from build123d import *

# Parameters (mm, degrees)
SKETCH1_R              = 6.35
SKETCH1_R_2            = 11.1125
BOSS_EXTRUDE1_DEPTH    = 6.35
F_10_CLEARANCE_HOLE1_D = 4.9784


with BuildPart() as part:
    # Sketch1 → Boss-Extrude1 (new body)
    with BuildSketch(Plane(origin=(0, 0, 0), x_dir=(0, 0, -1), z_dir=(1, 0, 0))):
        with BuildLine():
            Line((-25.748192037, 52.738776596), (-10.728413349, -2.896343085))
            ThreePointArc((-10.728413349, -2.896343085), (0, -11.1125), (10.728413349, -2.896343085))
            Line((10.728413349, -2.896343085), (25.748192037, 52.738776596))
            ThreePointArc((25.748192037, 52.738776596), (26.438543659, 56.183961041), (26.67, 59.69))
            Line((26.67, 59.69), (26.67, 100.96397257))
            Line((26.67, 100.96397257), (-26.67, 100.96397257))
            Line((-26.67, 100.96397257), (-26.67, 59.69))
            ThreePointArc((-26.67, 59.69), (-26.438543659, 56.183961041), (-25.748192037, 52.738776596))
        make_face()
        Circle(SKETCH1_R, mode=Mode.SUBTRACT)
        with Locations((0, 59.69)):
            Circle(SKETCH1_R_2, mode=Mode.SUBTRACT)
    extrude(amount=BOSS_EXTRUDE1_DEPTH)

    # #10 Clearance Hole1 (through all)
    with Locations(Plane.ZY):
        with Locations((20.32, 96.20147257), (-20.32, 96.20147257)):
            Hole(F_10_CLEARANCE_HOLE1_D / 2)


solid = part.part
Check sheet for the modelled part. Datum: model origin and axes. Units: mm. Give positions to 0.01 mm unless a question says otherwise; leave off trailing zeros. Loops run counter-clockwise (first coordinate to the right, second up) from the corner with the lowest first, then second, coordinate; pieces in that order, holes last. Notation, with made-up numbers: M 44,40 L 73,40 A29 ccw 73,78 Z; hole C 51,56 d7. An arc over 180 degrees is marked long. Use a Markdown table: item, result. Add a question column.
Q1. Sectioned sample at C-C, the plane x = 4.75. Give the number of separate pieces and of enclosed holes in the cut face, then the cut area to 3 significant figures.
Q2. Sectioned sample at B-B, the plane z = -5. Record the cut outline in (x, y).
Q3. Sectioned sample at D-D, the plane z = -20.32. Record the cut outline in (x, y), then the cut area to 3 significant figures.
Q4. Sectioned sample at A-A, the plane z = 9. Record the cut outline in (x, y), then the cut area to 3 significant figures.
Q5. Mould release check, pull along Z, two halves, no side actions. Record for faces 1 (the cylindrical face through (3.13, -11.11, 0.2)), 2 (the cylindrical face through (3.219, 93.993, -21.469)), 3 (the flat face through (3, 81, 26.67)), 4 (the cylindrical face through (3.131, 49.831, -5.128)): pulls with the +Z half, pulls with the -Z half, needs draft (parallel to the pull), parting line crosses it, or undercut.
Q6. Scan lines: line 1 along Y through (x, z) = (1, -4); line 2 along Z through (x, y) = (3, 95); line 3 along Z through (x, y) = (6, 23.5). Record each from-to range of solid material in increasing order. Write a range as [from, to].
Q7. Go/stop test with flat-tipped pins: pin 1 (4 mm diameter, centred on y = 96.2, z = 20.32, fed in from -X); pin 2 (1.5 mm diameter, centred on x = 5, z = 1.5, fed in from -Y); pin 3 (10 mm diameter, centred on y = 19, z = 17, fed in from +X); pin 4 (3 mm diameter, centred on x = 4.5, y = 55.5, fed in from +Z). Record where each tip stops, or that it passes through.
Verdict:
| question | item | result |
|---|---|---|
| 1 | separate pieces | 1 |
| 1 | enclosed holes | 4 |
| 1 | area | 4,170 mm^2 |
| 2 | outline | M 0,-9.92 L 6.35,-9.92 L 6.35,-3.91 L 0,-3.91 Z; M 0,3.91 L 6.35,3.91 L 6.35,49.77 L 0,49.77 Z; M 0,69.61 L 6.35,69.61 L 6.35,100.96 L 0,100.96 Z |
| 3 | outline | M 0,32.63 L 6.35,32.63 L 6.35,93.71 L 0,93.71 Z; M 0,98.69 L 6.35,98.69 L 6.35,100.96 L 0,100.96 Z |
| 3 | area | 402 mm^2 |
| 4 | outline | M 0,-6.52 L 6.35,-6.52 L 6.35,53.17 L 0,53.17 Z; M 0,66.21 L 6.35,66.21 L 6.35,100.96 L 0,100.96 Z |
| 4 | area | 600 mm^2 |
| 5 | face 1 | parting line crosses it |
| 5 | face 2 | undercut |
| 5 | face 3 | pulls with the +Z half |
| 5 | face 4 | undercut |
| 6 | line 1 | [-10.37, -4.93], [4.93, 49.32], [70.06, 100.96] |
| 6 | line 2 | [-26.67, -22.5], [-18.14, 18.14], [22.5, 26.67] |
| 6 | line 3 | [-17.85, 17.85] |
| 7 | pin 1 | through |
| 7 | pin 2 | y = -11.09 |
| 7 | pin 3 | x = 6.35 |
| 7 | pin 4 | z = 26.53 |
